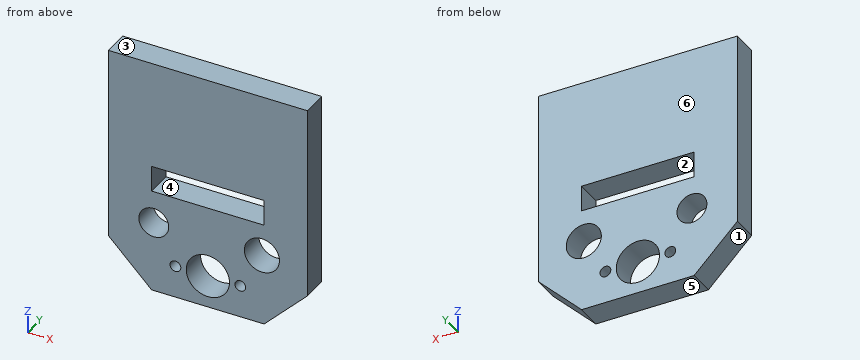
```python
from build123d import *

# Parameters (mm, degrees)
SKETCH1_W           = 92
SKETCH1_H           = 110
BOSS_EXTRUDE1_DEPTH = 12
CUT_EXTRUDE1_REACH  = 74.698
SKETCH2_R           = 10
SKETCH2_R_2         = 6.902314271
SKETCH2_R_3         = 8.115527509
SKETCH2_R_4         = 2.5
CUT_EXTRUDE2_REACH  = 74.698
SKETCH3_W           = 52
SKETCH3_H           = 12
CHAMFER1_SIZE       = 20


with BuildPart() as part:
    # Sketch1 → Boss-Extrude1 (new body)
    with BuildSketch(Plane(origin=(0, 0, 0), x_dir=(1, 0, 0), z_dir=(0, 1, 0))):
        Rectangle(SKETCH1_W, SKETCH1_H)
    extrude(amount=BOSS_EXTRUDE1_DEPTH)

    # Sketch2 → Cut-Extrude1 (cut, up to next)
    with BuildSketch(Plane(origin=(0, 12, 0), x_dir=(1, 0, 0), z_dir=(0, 1, 0)), mode=Mode.PRIVATE) as cut_extrude1_sk1:
        with Locations(Location((0, 40, 0), (0, 0, 270))):
            Circle(SKETCH2_R)
    cut_extrude1_tool1 = extrude(cut_extrude1_sk1.sketch, amount=-CUT_EXTRUDE1_REACH, mode=Mode.PRIVATE) & part.part
    # Sketch2 → Cut-Extrude1 (cut, up to next)
    with BuildSketch(Plane(origin=(0, 12, 0), x_dir=(1, 0, 0), z_dir=(0, 1, 0)), mode=Mode.PRIVATE) as cut_extrude1_sk2:
        with Locations(Location((-25, 22, 0), (0, 0, 270))):
            Circle(SKETCH2_R_2)
    cut_extrude1_tool2 = extrude(cut_extrude1_sk2.sketch, amount=-CUT_EXTRUDE1_REACH, mode=Mode.PRIVATE) & part.part
    # Sketch2 → Cut-Extrude1 (cut, up to next)
    with BuildSketch(Plane(origin=(0, 12, 0), x_dir=(1, 0, 0), z_dir=(0, 1, 0)), mode=Mode.PRIVATE) as cut_extrude1_sk3:
        with Locations(Location((25, 22, 0), (0, 0, 270))):
            Circle(SKETCH2_R_3)
    cut_extrude1_tool3 = extrude(cut_extrude1_sk3.sketch, amount=-CUT_EXTRUDE1_REACH, mode=Mode.PRIVATE) & part.part
    # Sketch2 → Cut-Extrude1 (cut, up to next)
    with BuildSketch(Plane(origin=(0, 12, 0), x_dir=(1, 0, 0), z_dir=(0, 1, 0)), mode=Mode.PRIVATE) as cut_extrude1_sk4:
        with Locations(Location((-15, 40, 0), (0, 0, 270))):
            Circle(SKETCH2_R_4)
    cut_extrude1_tool4 = extrude(cut_extrude1_sk4.sketch, amount=-CUT_EXTRUDE1_REACH, mode=Mode.PRIVATE) & part.part
    # Sketch2 → Cut-Extrude1 (cut, up to next)
    with BuildSketch(Plane(origin=(0, 12, 0), x_dir=(1, 0, 0), z_dir=(0, 1, 0)), mode=Mode.PRIVATE) as cut_extrude1_sk5:
        with Locations(Location((15, 40, 0), (0, 0, 270))):
            Circle(SKETCH2_R_4)
    cut_extrude1_tool5 = extrude(cut_extrude1_sk5.sketch, amount=-CUT_EXTRUDE1_REACH, mode=Mode.PRIVATE) & part.part
    add(cut_extrude1_tool1.solids().sort_by_distance((0, 12, -40))[0], mode=Mode.SUBTRACT)
    add(cut_extrude1_tool2.solids().sort_by_distance((-25, 12, -22))[0], mode=Mode.SUBTRACT)
    add(cut_extrude1_tool3.solids().sort_by_distance((25, 12, -22))[0], mode=Mode.SUBTRACT)
    add(cut_extrude1_tool4.solids().sort_by_distance((-15, 12, -40))[0], mode=Mode.SUBTRACT)
    add(cut_extrude1_tool5.solids().sort_by_distance((15, 12, -40))[0], mode=Mode.SUBTRACT)

    # Sketch3 → Cut-Extrude2 (cut, up to next)
    with BuildSketch(Plane(origin=(0, 12, 0), x_dir=(1, 0, 0), z_dir=(0, 1, 0)), mode=Mode.PRIVATE) as cut_extrude2_sk1:
        with Locations((0, 1)):
            Rectangle(SKETCH3_W, SKETCH3_H)
    cut_extrude2_tool1 = extrude(cut_extrude2_sk1.sketch, amount=-CUT_EXTRUDE2_REACH, mode=Mode.PRIVATE) & part.part
    add(cut_extrude2_tool1.solids().sort_by_distance((0, 12, -1))[0], mode=Mode.SUBTRACT)

    # Chamfer1
    chamfer1_edges = [part.edges().sort_by_distance(p)[0] for p in [
        (-46, 6, -55),
        (46, 6, -55),
    ]]
    chamfer(chamfer1_edges, length=CHAMFER1_SIZE)


solid = part.part
```
For this review, take the finished solid that the model builds, in its own axes (mm). Face numbers are marked on the shaded views. A direction names the side the tool comes from. Coordinates: 2 decimals unless noted, no trailing zeros. Write each loop counter-clockwise with the first axis right and the second up, starting at its lowest first coordinate (ties: lowest second). Pieces come first, ordered by that corner, then holes. Notation, with made-up numbers: (21.25, -22.5) -> (37.25, -22.5) arc R29 cw to (37.25, 13.5) -> close; hole circle Ø3 at (64.5, -5.75). An arc over 180 degrees is marked (long way). Put each result on its own line as item: value.
Q1. The part is to be moulded in two halves that separate along Z. For the marked faces 3, 4, 5 and 6, say which applies: +Z half, -Z half, draft (parallel to the pull), parting line (faces both ways), or undercut.
From the geometry:
face 3: +Z half
face 4: undercut
face 5: -Z half
face 6: draft
Q2. Take a section at A-A, the plane x = 0. State the section outline as (y, z) points.
From the geometry:
outline: (0, -55) -> (12, -55) -> (12, -50) -> (0, -50) -> close; (0, -30) -> (12, -30) -> (12, -7) -> (0, -7) -> close; (0, 5) -> (12, 5) -> (12, 55) -> (0, 55) -> close
Q3. Take a section at B-B, the plane z = -40. State the section outline as (x, y) points, then the cut area to 3 significant figures.
From the geometry:
outline: (-41, 0) -> (-17.5, 0) -> (-17.5, 12) -> (-41, 12) -> close; (-12.5, 0) -> (-10, 0) -> (-10, 12) -> (-12.5, 12) -> close; (10, 0) -> (12.5, 0) -> (12.5, 12) -> (10, 12) -> close; (17.5, 0) -> (41, 0) -> (41, 12) -> (17.5, 12) -> close
area: 624 mm2
Q4. Tool access review of the marked faces 1 and 2: name each direction out of +Z, -Z, +X, -X, +Y, -Y from which nothing blocks a thin tool from reaching the whole face with its end or side.
From the geometry:
face 1: -Z, -X, +Y, -Y
face 2: +Y, -Y
Q5. Take a section at D-D, the plane z = -1.5. State the section outline as (x, y) points, then the cut area to 3 significant figures.
From the geometry:
outline: (-46, 0) -> (-26, 0) -> (-26, 12) -> (-46, 12) -> close; (26, 0) -> (46, 0) -> (46, 12) -> (26, 12) -> close
area: 480 mm2
Q6. Take a section at C-C, the plane y = 10.5. State the section outline as (x, z) points, then the cut area to 3 significant figures.
From the geometry:
outline: (-46, -35) -> (-26, -55) -> (26, -55) -> (46, -35) -> (46, 55) -> (-46, 55) -> close; hole circle Ø13.8 at (-25, -22); hole (-26, -7) -> (26, -7) -> (26, 5) -> (-26, 5) -> close; hole circle Ø5 at (-15, -40); hole circle Ø20 at (0, -40); hole circle Ø5 at (15, -40); hole circle Ø16.23 at (25, -22)
area: 8,390 mm2
Q7. Clearance check with a flat-ended pin moving along its axis: pin 1 Ø4.5 at (x, z) = (15, -40) entering from +Y. State where the tip first meets the part, or that it passes through.
From the geometry:
pin 1: passes through
Q8. Wall thickness on L1, parallel to X at y = 8.75, z = -22; L2, parallel to X at y = 7.5, z = -40; L3, parallel to Z at x = -17, y = 1: over which ranges is each line inside the solid? List them lowest first.
From the geometry:
L1: x = -46 to -31.9, -18.1 to 16.88, 33.12 to 46
L2: x = -41 to -17.5, -12.5 to -10, 10 to 12.5, 17.5 to 41
L3: z = -55 to -41.5, -38.5 to -7, 5 to 55
